```python
from build123d import *

# Parameters (mm, degrees)
PASSIVE_ARM_START = 8
PROFILE_1_R       = 5.05
PASSIVE_ARM_DEPTH = 10


with BuildPart() as part:
    # Profile_1 → Passive_arm (new body)
    with BuildSketch(Plane.XY.offset(PASSIVE_ARM_START)):
        Polygon((9.146165735, 6.111272563), (6.111272563, 9.146165735), (2.145993542, 10.788638084), (-112.145993542, 10.788638084), (-116.111272563, 9.146165735), (-119.146165735, 6.111272563), (-120.788638084, 2.145993542), (-120.788638084, -2.145993542), (-119.146165735, -6.111272563), (-116.111272563, -9.146165735), (-112.145993542, -10.788638084), (2.145993542, -10.788638084), (6.111272563, -9.146165735), (9.146165735, -6.111272563), (10.788638084, -2.145993542), (10.788638084, 2.145993542), align=None)
        Circle(PROFILE_1_R, mode=Mode.SUBTRACT)
        with Locations((-110, 0)):
            Circle(PROFILE_1_R, mode=Mode.SUBTRACT)
    extrude(amount=PASSIVE_ARM_DEPTH)


solid = part.part
```
Part model, mm, in its own coordinate system. Round coordinates to 2 decimals unless told otherwise and drop trailing zeros. Write each loop counter-clockwise with the first axis right and the second up, starting at its lowest first coordinate (ties: lowest second). Pieces come first, ordered by that corner, then holes.
Item 1: Drop a flat-ended pin along its axis: pin 1 Ø4 at (y, z) = (7.5, 15) entering from +X. Give the stop position or say it passes through.
Results:
pin 1: stops at x = 9.4
Item 2: Cut at D-D, the plane x = -3. Give the cut face in (y, z).
Results:
outline: (-10.79, 8) - (-4.06, 8) - (-4.06, 18) - (-10.79, 18) - close; (4.06, 8) - (10.79, 8) - (10.79, 18) - (4.06, 18) - close
Item 3: Cut at B-B, the plane x = -110. Give the cut face in (y, z).
Results:
outline: (-10.79, 8) - (-5.05, 8) - (-5.05, 18) - (-10.79, 18) - close; (5.05, 8) - (10.79, 8) - (10.79, 18) - (5.05, 18) - close
Item 4: Cut at C-C, the plane z = 11.25. Give the cut face in (x, y).
Results:
outline: (-120.79, -2.15) - (-119.15, -6.11) - (-116.11, -9.15) - (-112.15, -10.79) - (2.15, -10.79) - (6.11, -9.15) - (9.15, -6.11) - (10.79, -2.15) - (10.79, 2.15) - (9.15, 6.11) - (6.11, 9.15) - (2.15, 10.79) - (-112.15, 10.79) - (-116.11, 9.15) - (-119.15, 6.11) - (-120.79, 2.15) - close; hole circle Ø10.1 at (-110, 0); hole circle Ø10.1 at (0, 0)
Item 5: Cut at A-A, the plane y = 0. Give the cut face in (x, z).
Results:
outline: (-120.79, 8) - (-115.05, 8) - (-115.05, 18) - (-120.79, 18) - close; (-104.95, 8) - (-5.05, 8) - (-5.05, 18) - (-104.95, 18) - close; (5.05, 8) - (10.79, 8) - (10.79, 18) - (5.05, 18) - close
Item 6: Probe L1, parallel to X at y = 0.5, z = 16; L2, parallel to Y at x = -110, z = 15.5; L3, parallel to X at y = 2.5, z = 13. List the from-to ranges inside material, lowest first.
Results:
L1: x = -120.79 to -115.03, -104.97 to -5.03, 5.03 to 10.79
L2: y = -10.79 to -5.05, 5.05 to 10.79
L3: x = -120.64 to -114.39, -105.61 to -4.39, 4.39 to 10.64
Item 7: Two-plate mould, pull along X, no slides. Class faces 1 (the flat face through (10.789, 0, 13)), 2 (the flat face through (-54, 10.789, 13)), 3 (the cylindrical face through (4.817, 1.517, 12.93)): +X half, -X half, draft (parallel to the pull), parting line (faces both ways), or undercut.
Results:
face 1: +X half
face 2: draft
face 3: undercut
